```python
from build123d import *

# Parameters (mm, degrees)
F0_R     = 127
F0_R_2   = 12.7
F1_DEPTH = 19.05


with BuildPart() as f1:
    # F0 (on Top) → F1 (new body, symmetric)
    with BuildSketch(Plane.XY):
        Circle(F0_R)
        with BuildLine():
            ThreePointArc((-82.161109, 70.019674), (-48.159661, 96.61185), (-6.457917, 107.75666))
            Line((-6.457917, 107.75666), (6.457917, 107.75666))
            ThreePointArc((6.457917, 107.75666), (47.964828, 96.708726), (81.878172, 70.350319))
            ThreePointArc((81.878172, 70.350319), (100.263633, 40.00508), (107.81793, 5.338218))
            ThreePointArc((107.81793, 5.338218), (107.95, 0), (107.81793, -5.338218))
            ThreePointArc((107.81793, -5.338218), (101.460657, -36.86377), (86.098285, -65.117492))
            ThreePointArc((86.098285, -65.117492), (50.952795, -95.168352), (6.457917, -107.75666))
            ThreePointArc((6.457917, -107.75666), (0, -107.95), (-6.457917, -107.75666))
            ThreePointArc((-6.457917, -107.75666), (-44.708732, -98.256459), (-76.999847, -75.658616))
            ThreePointArc((-76.999847, -75.658616), (-98.871847, -43.330824), (-107.81793, -5.338218))
            ThreePointArc((-107.81793, -5.338218), (-107.95, 0), (-107.81793, 5.338218))
            ThreePointArc((-107.81793, 5.338218), (-100.344065, 39.802903), (-82.161109, 70.019674))
        make_face(mode=Mode.SUBTRACT)
        with BuildLine():
            ThreePointArc((-6.457917, 43.978379), (-21.521062, 38.892755), (-33.831045, 28.83163))
            ThreePointArc((-33.831045, 28.83163), (-40.711172, 17.843849), (-44.128289, 5.338218))
            Line((-44.128289, 5.338218), (-44.128289, -5.338218))
            ThreePointArc((-44.128289, -5.338218), (-40.053849, -19.274119), (-31.705819, -31.153548))
            ThreePointArc((-31.705819, -31.153548), (-20.130494, -39.630364), (-6.457917, -43.978379))
            Line((-6.457917, -43.978379), (6.457917, -43.978379))
            ThreePointArc((6.457917, -43.978379), (22.644581, -38.249516), (35.452235, -26.813085))
            ThreePointArc((35.452235, -26.813085), (41.213559, -16.650677), (44.128289, -5.338218))
            Line((44.128289, -5.338218), (44.128289, 5.338218))
            ThreePointArc((44.128289, 5.338218), (40.675123, 17.925872), (33.714542, 28.967779))
            ThreePointArc((33.714542, 28.967779), (21.442625, 38.936055), (6.457917, 43.978379))
            Line((6.457917, 43.978379), (-6.457917, 43.978379))
        make_face()
        Circle(F0_R_2, mode=Mode.SUBTRACT)
        with BuildLine():
            Line((6.457917, 107.75666), (-6.457917, 107.75666))
            ThreePointArc((-6.457917, 107.75666), (-48.159661, 96.61185), (-82.161109, 70.019674))
            Line((-82.161109, 70.019674), (-33.831045, 28.83163))
            ThreePointArc((-33.831045, 28.83163), (-21.521062, 38.892755), (-6.457917, 43.978379))
            Line((-6.457917, 43.978379), (6.457917, 43.978379))
            ThreePointArc((6.457917, 43.978379), (21.442625, 38.936055), (33.714542, 28.967779))
            Line((33.714542, 28.967779), (81.878172, 70.350319))
            ThreePointArc((81.878172, 70.350319), (47.964828, 96.708726), (6.457917, 107.75666))
        make_face()
        with BuildLine():
            Line((-31.705819, -31.153548), (-76.999847, -75.658616))
            ThreePointArc((-76.999847, -75.658616), (-44.708732, -98.256459), (-6.457917, -107.75666))
            Line((-6.457917, -107.75666), (6.457917, -107.75666))
            ThreePointArc((6.457917, -107.75666), (50.952795, -95.168352), (86.098285, -65.117492))
            Line((86.098285, -65.117492), (35.452235, -26.813085))
            ThreePointArc((35.452235, -26.813085), (22.644581, -38.249516), (6.457917, -43.978379))
            ThreePointArc((6.457917, -43.978379), (0, -44.45), (-6.457917, -43.978379))
            ThreePointArc((-6.457917, -43.978379), (-20.130494, -39.630364), (-31.705819, -31.153548))
        make_face()
    extrude(amount=F1_DEPTH, both=True)


solid = f1.part
```
Read the model definition and answer for the solid it produces. Units are mm, in the model's axes. A direction names the side the tool comes from. Coordinates: 2 decimals unless noted, no trailing zeros. Loops run counter-clockwise (first coordinate to the right, second up) from the corner with the lowest first, then second, coordinate; pieces in that order, holes last.
(1) The part is cut by section A-A (x = 0). Determine the outline of the cut face in (y, z), and give its area (3 significant figures).
Solution:
outline: (-127, -19.05) - (-107.95, -19.05) - (-107.95, 19.05) - (-127, 19.05) - close; (-107.76, -19.05) - (-44.45, -19.05) - (-44.45, 19.05) - (-107.76, 19.05) - close; (-43.98, -19.05) - (-12.7, -19.05) - (-12.7, 19.05) - (-43.98, 19.05) - close; (12.7, -19.05) - (127, -19.05) - (127, 19.05) - (12.7, 19.05) - close
area: 8,680 mm2
(2) Consider line 1 along X through (y, z) = (47, 12); line 2 along X through (y, z) = (-58, -2); line 3 along Y through (x, z) = (-72.5, -1.5). Determine where each line is inside the solid, lowest interval first.
Solution:
line 1: x = -117.98 to -97.18, -55.15 to 54.7, 97.18 to 117.98
line 2: x = -112.98 to -91.05, -59.03 to 76.69, 91.05 to 112.98
line 3: y = -104.27 to -71.24, 61.79 to 104.27
(3) A tool of negligible diameter and unlimited length cuts with its end or side. For faces 1 (the face through (41.152, -16.803, 0.267)), 2 (the face through (26, 2, -19.05)), from which of +Z, -Z, +X, -X, +Y, -Y can it reach the whole face along a straight path? Write none if from no direction.
Solution:
face 1: +Z, -Z
face 2: -Z, +X, -X, +Y, -Y
(4) The part is cut by section B-B (y = 0). Determine the outline of the cut face in (x, z).
Solution:
outline: (-127, -19.05) - (-107.95, -19.05) - (-107.95, 19.05) - (-127, 19.05) - close; (-44.13, -19.05) - (-12.7, -19.05) - (-12.7, 19.05) - (-44.13, 19.05) - close; (12.7, -19.05) - (44.13, -19.05) - (44.13, 19.05) - (12.7, 19.05) - close; (107.95, -19.05) - (127, -19.05) - (127, 19.05) - (107.95, 19.05) - close
(5) The part is cut by section D-D (x = 40). Determine the outline of the cut face in (y, z), and give its area (3 significant figures).
Solution:
outline: (-120.54, -19.05) - (-30.25, -19.05) - (-30.25, 19.05) - (-120.54, 19.05) - close; (-19.39, -19.05) - (19.39, -19.05) - (19.39, 19.05) - (-19.39, 19.05) - close; (34.37, -19.05) - (120.54, -19.05) - (120.54, 19.05) - (34.37, 19.05) - close
area: 8,200 mm2
(6) Flat-ended cylindrical pins translate along their axes: pin 1 Ø12 at (y, z) = (-66, -7.5) entering from -X; pin 2 Ø2 at (x, z) = (60, 11.5) entering from -Y; pin 3 Ø12 at (x, z) = (-14.5, 0) entering from -Y. Find the tip coordinate at first contact, or state that the pin passes through.
Solution:
pin 1: stops at x = -111.93
pin 2: stops at y = -112.46
pin 3: stops at y = -126.72
(7) The mould has two halves that part along Y. Classify faces 3 (the face through (40.75, 17.76, 0.27)), 4 (the face through (26, 2, 19.05)), 5 (the face through (-27.53, -123.98, 0.27)): released by +Y, released by -Y, zero draft, split by the parting line, or undercut.
Solution:
face 3: undercut
face 4: zero draft
face 5: split by the parting line
(8) The part is cut by section C-C (z = 11.5). Determine the outline of the cut face in (x, y).
Solution:
outline: circle Ø254 at (0, 0); hole (-107.82, -5.34) arc R107.95 ccw to (-77, -75.66) - (-31.71, -31.15) arc R44.45 cw to (-44.13, -5.34) - (-44.13, 5.34) arc R44.45 cw to (-33.83, 28.83) - (-82.16, 70.02) arc R107.95 ccw to (-107.82, 5.34) arc R107.95 ccw to start; hole circle Ø25.4 at (0, 0); hole (-6.46, -107.76) arc R107.95 ccw to (6.46, -107.76) - close; hole (-6.46, -43.98) arc R44.45 ccw to (6.46, -43.98) - close; hole (33.71, 28.97) arc R44.45 cw to (44.13, 5.34) - (44.13, -5.34) arc R44.45 cw to (35.45, -26.81) - (86.1, -65.12) arc R107.95 ccw to (107.82, -5.34) arc R107.95 ccw to (107.82, 5.34) arc R107.95 ccw to (81.88, 70.35) - close
